Input: part model. Units: mm. Frame: model coordinates. Face numbers are marked on the shaded views. A direction names the side the tool comes from. Give positions to 0.01 mm unless a question says otherwise; leave off trailing zeros. Loops run counter-clockwise (first coordinate to the right, second up) from the corner with the lowest first, then second, coordinate; pieces in that order, holes last. Notation, with made-up numbers: (18, 88) -> (53, 88) arc R5 cw to (53, 95) -> close; hole circle Ø5 at (89.25, -19). An arc over 180 degrees is marked (long way). Answer as a JSON object with one key per item and string values.
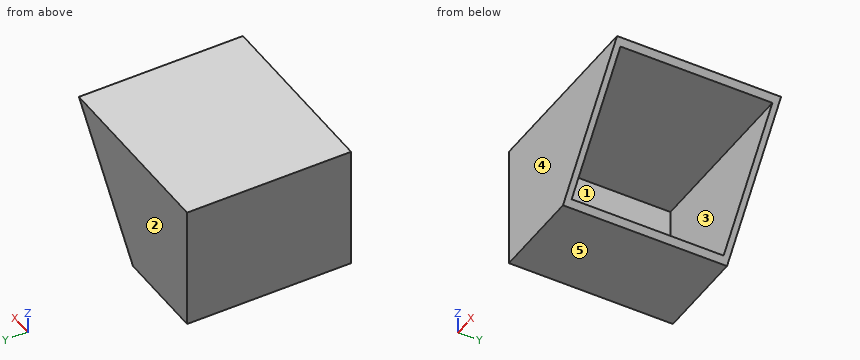
```python
from build123d import *

# Parameters (mm, degrees)
F0_W     = 60.931796
F0_H     = 54.4
F0_W_2   = 56.931796
F0_H_2   = 50.4
F1_DEPTH = 41
F3_DEPTH = 54.401
F4_T     = -2


with BuildPart() as f1:
    # F0 (on Top) → F1 (new body)
    with BuildSketch(Plane.XY):
        Rectangle(F0_W, F0_H)
        Rectangle(F0_W_2, F0_H_2, mode=Mode.SUBTRACT)
        Rectangle(F0_W_2, F0_H_2)
    extrude(amount=F1_DEPTH)

    # F2 (on face) → F3 (cut, through all)
    with BuildSketch(Plane.XZ.offset(27.2)):
        Polygon((30.465898, 0), (30.465898, 41), (0, 0), align=None)
    extrude(amount=-F3_DEPTH, mode=Mode.SUBTRACT)

    # F4
    f4_openings = [f1.faces().sort_by_distance(p)[0] for p in [
        (15.232949, 0, 20.5),
    ]]
    offset(amount=F4_T, openings=f4_openings)


solid = f1.part
```
Q1. Access query for the marked faces 1 and 2. Directions: +Z, -Z, +X, -X, +Y, -Y. A direction counts if a zero-diameter tool reaches every point of the face in a straight line with its end or side. Return the directions, or none.
Evaluation:
{"face 1": "+X", "face 2": "+Z, -Z, +X, -X, +Y"}
Q2. Section C-C, the plane y = -17. Return the cut outline in (x, z), then the cut area to 3 significant figures.
Evaluation:
{"outline": "(-30.47, 0) -> (0, 0) -> (1.49, 2) -> (-28.47, 2) -> (-28.47, 39) -> (28.98, 39) -> (30.47, 41) -> (-30.47, 41) -> close", "area": "257 mm2"}
Q3. Section A-A, the plane x = -3. Return the cut outline in (y, z), then the cut area to 3 significant figures.
Evaluation:
{"outline": "(-27.2, 0) -> (27.2, 0) -> (27.2, 41) -> (-27.2, 41) -> close; hole (-25.2, 2) -> (25.2, 2) -> (25.2, 39) -> (-25.2, 39) -> close", "area": "366 mm2"}
Q4. Ray query, line 1 along Y through (x, z) = (-16, 12); line 2 along Z through (x, y) = (-16, -11); line 3 along Z through (x, y) = (4.5, -9). Return the intervals inside material, ascending.
Evaluation:
{"line 1": "y = -27.2 to -25.2, 25.2 to 27.2", "line 2": "z = 0 to 2, 39 to 41", "line 3": "z = 39 to 41"}
Q5. Section B-B, the plane z = 31. Return the cut outline in (x, y), then the cut area to 3 significant figures.
Evaluation:
{"outline": "(-30.47, -27.2) -> (23.04, -27.2) -> (23.04, -25.2) -> (-28.47, -25.2) -> (-28.47, 25.2) -> (23.04, 25.2) -> (23.04, 27.2) -> (-30.47, 27.2) -> close", "area": "315 mm2"}
Q6. Pin query (flat end, axial travel): pin 1 (4 mm diameter, centred on y = 14, z = 24.5, fed in from +X); pin 2 (10 mm diameter, centred on x = 24.5, z = 20, fed in from -Y). Return the tip coordinate at first contact, or that it passes through.
Evaluation:
{"pin 1": "stops at x = -28.47", "pin 2": "passes through"}
Q7. Draft query along Y for the marked faces 3, 4 and 5. Return one class per face: +Y half, -Y half, draft (parallel to the pull), parting line (faces both ways), or undercut.
Evaluation:
{"face 3": "undercut", "face 4": "-Y half", "face 5": "draft"}
